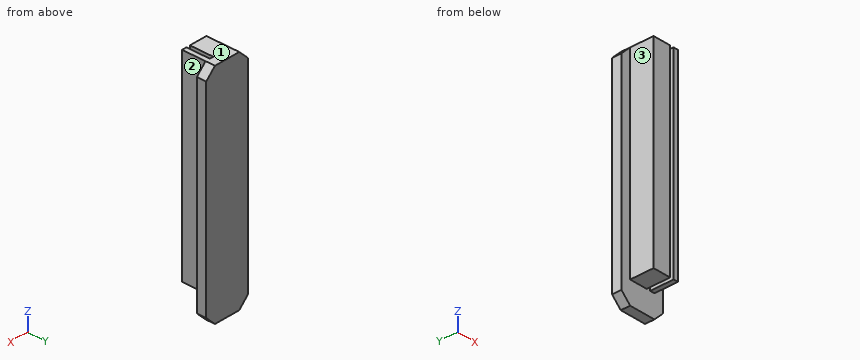
Autodesk Inventor part; units mm, degrees
ref_plane "YZ Plane" through (0, 0, 0) normal (1, 0, 0) x (0, 1, 0)
ref_plane "XZ Plane" through (0, 0, 0) normal (0, 1, 0) x (-1, 0, 0)
ref_plane "XY Plane" through (0, 0, 0) normal (0, 0, 1) x (1, 0, 0)
sketch "Sketch1" plane through (0, 0, 0) normal (0, 1, 0) x (-1, 0, 0)
  line L0 (45.4816, -24) -> (64.4816, -24)
  line L1 (64.4816, -224) -> (45.4816, -224)
  line L2 (64.4816, -24) -> (52.9072, -24)
  line L3 (45.4816, -51) -> (64.4816, -51)
  line L4 (64.4816, -50.2724) -> (64.4816, -24)
  line L5 (64.4816, -69) -> (45.4816, -69)
  line L6 (45.4816, -51) -> (45.4816, -24)
  line L7 (64.4816, -24) -> (64.4816, -51)
  line L8 (64.4816, -154) -> (45.4816, -154)
  line L9 (64.4816, -204) -> (45.4816, -204)
  line L10 (45.4816, -224) -> (45.4816, -204)
  line L11 (45.4816, -154) -> (45.4816, -69)
  line L12 (64.4816, -69) -> (64.4816, -154)
  line L13 (64.4816, -204) -> (64.4816, -224)
  line L14 (41.4816, -24) -> (36.4816, -24)
  line L15 (36.4816, -24) -> (36.4816, -224)
  line L16 (36.4816, -224) -> (41.4816, -224)
  line L17 (41.4816, -224) -> (41.4816, -24)
  point P0 (0, 0)
  dimension "d0" = 200
  dimension "d1" = 19
  dimension "d7" = 27
  dimension "d9" = 45
  dimension "d11" = 85
  dimension "d12" = 20
  dimension "d13" = 4
  dimension "d14" = 19
  dimension "d15" = 5
extrude "Extrusion2" add sketch "Sketch1" along normal blind 11
sketch "Sketch2" plane through (0, 11, 0) normal (0, 1, 0) x (1, 0, 0)
  line L0 (-64.4816, 224) -> (-36.4816, 224)
  line L1 (-36.4816, 224) -> (-36.4816, 24)
  line L2 (-36.4816, 24) -> (-64.4816, 24)
  line L3 (-64.4816, 24) -> (-64.4816, 224)
  point P0 (0, 0)
extrude "Extrusion3" add sketch "Sketch2" along normal blind 3
sketch "Sketch3" plane through (0, 0, 0) normal (0, -1, 0) x (1, 0, 0)
  line L0 (-19.3539, -51.0239) -> (-76.8291, -51.0239)
  line L1 (-76.8291, -51.0239) -> (-76.8291, -110.8451)
  line L2 (-76.8291, -110.8451) -> (-19.3539, -110.8451)
  line L3 (-19.3539, -110.8451) -> (-19.3539, -51.0239)
  line L4 (-25.2187, -135.4773) -> (-86.9948, -135.4773)
  line L5 (-86.9948, -135.4773) -> (-86.9948, -203.9002)
  line L6 (-86.9948, -203.9002) -> (-25.2187, -203.9002)
  line L7 (-25.2187, -203.9002) -> (-25.2187, -135.4773)
  point P0 (0, 0)
extrude "Extrusion4" cut sketch "Sketch3" against normal up to surface (11 mm away)
sketch "Sketch4" plane through (0, 14, 0) normal (0, 1, 0) x (1, 0, 0)
  line L0 (-64.4816, 24) -> (-36.4816, 24)
  line L1 (-26.4816, 34) -> (-26.4816, 251)
  line L2 (-36.4816, 261) -> (-64.4816, 261)
  line L3 (-74.4816, 251) -> (-74.4816, 34)
  line L4 (-64.4816, 224) -> (-64.4816, 24)
  line L5 (-36.4816, 24) -> (-36.4816, 224)
  line L6 (-36.4816, 224) -> (-64.4816, 224)
  line L7 (-64.4816, 24) -> (-74.4816, 34)
  line L8 (-36.4816, 24) -> (-26.4816, 34)
  line L9 (-64.4816, 261) -> (-74.4816, 251)
  line L10 (-36.4816, 261) -> (-26.4816, 251)
  point P0 (0, 0)
  point P1 (-74.4816, 24)
  point P2 (-26.4816, 261)
  point P3 (-26.4816, 24)
  point P4 (-74.4816, 261)
  dimension "d22" = 10
  dimension "d23" = 10
  dimension "d24" = 37
  dimension "d31" = 10
  dimension "d32" = 10
  dimension "d33" = 10
  dimension "d34" = 10
  dimension "d35" = 10
  dimension "d36" = 10
  dimension "d37" = 10
  dimension "d38" = 10
extrude "Extrusion5" add sketch "Sketch4" along normal blind 21
sketch "Sketch5" plane through (-45.4816, 0, -224) normal (0, 0, -1) x (-1, 0, 0)
  line L0 (-9, 0) -> (-4, 0)
  line L1 (-4, 0) -> (-4, 11)
  line L2 (0, 11) -> (-4, 11)
  line L3 (0, 0) -> (0, 11)
  line L4 (19, 0) -> (0, 0)
  line L5 (19, 0) -> (19, 14)
  line L6 (-9, 14) -> (19, 14)
  line L7 (-9, 0) -> (-9, 14)
  point P0 (-45.4816, 0)
extrude "Extrusion6" add sketch "Sketch5" along normal blind 13
sketch "Sketch6" plane through (0, 11, 0) normal (0, -1, 0) x (1, 0, 0)
  line L0 (-41.4816, -51.0239) -> (-41.4816, -24)
  line L1 (-41.4816, -24) -> (-45.4816, -24)
  line L2 (-45.4816, -24) -> (-45.4816, -51)
  line L3 (-45.4816, -51) -> (-64.4816, -51)
  line L4 (-64.4816, -110.8451) -> (-64.4816, -51)
  line L5 (-64.4816, -110.8451) -> (-45.4816, -110.8451)
  line L6 (-45.4816, -110.8451) -> (-45.4816, -135.4773)
  line L7 (-45.4816, -135.4773) -> (-64.4816, -135.4773)
  line L8 (-64.4816, -204) -> (-64.4816, -135.4773)
  line L9 (-64.4816, -204) -> (-45.4816, -204)
  line L10 (-45.4816, -204) -> (-45.4816, -237)
  line L11 (-41.4816, -237) -> (-45.4816, -237)
  line L12 (-41.4816, -203.9002) -> (-41.4816, -237)
  line L13 (-41.4816, -203.9002) -> (-36.4816, -203.9002)
  line L14 (-36.4816, -135.4773) -> (-36.4816, -203.9002)
  line L15 (-36.4816, -135.4773) -> (-41.4816, -135.4773)
  line L16 (-41.4816, -135.4773) -> (-41.4816, -110.8451)
  line L17 (-41.4816, -110.8451) -> (-36.4816, -110.8451)
  line L18 (-36.4816, -51.0239) -> (-36.4816, -110.8451)
  line L19 (-36.4816, -51.0239) -> (-41.4816, -51.0239)
  point P0 (0, 0)
extrude "Extrusion7" cut sketch "Sketch6" against normal up to surface (3 mm away)
sketch "Sketch7" plane through (0, 14, 0) normal (0, -1, 0) x (1, 0, 0)
  line L0 (-36.4816, -110.8451) -> (-36.4816, -135.4773)
  line L1 (-41.4816, -135.4773) -> (-36.4816, -135.4773)
  line L2 (-41.4816, -110.8451) -> (-41.4816, -135.4773)
  line L3 (-36.4816, -110.8451) -> (-41.4816, -110.8451)
  line L4 (-41.4816, -51.0239) -> (-36.4816, -51.0239)
  line L5 (-41.4816, -24) -> (-41.4816, -51.0239)
  line L6 (-45.4816, -24) -> (-41.4816, -24)
  line L7 (-45.4816, -51) -> (-45.4816, -24)
  line L8 (-64.4816, -51) -> (-45.4816, -51)
  line L9 (-64.4816, -51) -> (-64.4816, -24)
  line L10 (-64.4816, -24) -> (-74.4816, -34)
  line L11 (-74.4816, -34) -> (-74.4816, -251)
  line L12 (-74.4816, -251) -> (-64.4816, -261)
  line L13 (-64.4816, -261) -> (-36.4816, -261)
  line L14 (-36.4816, -261) -> (-26.4816, -251)
  line L15 (-26.4816, -251) -> (-26.4816, -34)
  line L16 (-26.4816, -34) -> (-36.4816, -24)
  line L17 (-36.4816, -24) -> (-36.4816, -51.0239)
  line L18 (-36.4816, -203.9002) -> (-36.4816, -237)
  line L19 (-36.4816, -237) -> (-41.4816, -237)
  line L20 (-41.4816, -203.9002) -> (-41.4816, -237)
  line L21 (-36.4816, -203.9002) -> (-41.4816, -203.9002)
  line L22 (-45.4816, -110.8451) -> (-64.4816, -110.8451)
  line L23 (-45.4816, -135.4773) -> (-45.4816, -110.8451)
  line L24 (-64.4816, -135.4773) -> (-45.4816, -135.4773)
  line L25 (-64.4816, -135.4773) -> (-64.4816, -110.8451)
  line L26 (-45.4816, -204) -> (-64.4816, -204)
  line L27 (-45.4816, -237) -> (-45.4816, -204)
  line L28 (-45.4816, -237) -> (-64.4816, -237)
  line L29 (-64.4816, -237) -> (-64.4816, -204)
  point P0 (0, 0)
extrude "Extrusion8" cut sketch "Sketch7" against normal blind 11
sketch "Sketch8" plane through (-64.4816, 0, -204) normal (0, 0, 1) x (1, 0, 0)
  line L0 (0, 0) -> (0, 25)
  line L1 (19, 0) -> (0, 0)
  line L2 (19, 0) -> (19, 25)
  line L3 (19, 25) -> (0, 25)
  line L4 (0, 0) -> (0, 25)
  line L5 (23, 0) -> (23, 25)
  line L6 (28, 0) -> (23, 0)
  line L7 (28, 25) -> (28, 0)
  line L8 (28, 25) -> (23, 25)
  point P0 (64.4816, 0)
extrude "Extrusion9" add sketch "Sketch8" along normal up to surface (180 mm away)
properties part number "cut platform"
Source: CAD feature listing. Evaluate the final solid. Frame: model axes, mm. Face numbers are marked on the shaded views. A direction names the side the tool comes from. Give positions to 0.01 mm unless a question says otherwise; leave off trailing zeros. Loops run counter-clockwise (first coordinate to the right, second up) from the corner with the lowest first, then second, coordinate; pieces in that order, holes last. Notation, with made-up numbers: (82.25, -28) -> (116.25, -28) arc R15 cw to (116.25, -24) -> close; hole circle Ø7 at (-39, 27). An arc over 180 degrees is marked (long way). Use a Markdown table: item, result. Add a question column.
1) First-contact query: pin 1 (8 mm diameter, centred on y = 4, z = -67, fed in from +X); pin 2 (9.5 mm diameter, centred on x = -59, y = 9, fed in from -Z); pin 3 (10 mm diameter, centred on x = -63, y = 21, fed in from -Z); pin 4 (2 mm diameter, centred on y = 13, z = -82, fed in from -X). Flat tips, straight axial feed; report the tip coordinate or a pass-through.
2) Section query D-D, the plane y = 30. Return the cut outline in (x, z), then the cut area to 3 significant figures.
3) Line query: line 1 along X through (y, z) = (6, -60); line 2 along Y through (x, z) = (-40, -250); line 3 along Z through (x, y) = (-47.5, 22.5). Output: solid intervals per line, ascending. Write a range as [from, to].
4) Reachability of the marked faces 1, 2 and 3 from +Z, -Z, +X, -X, +Y, -Y: full face, straight path, thin tool, end or side. Return the list, or none.
5) Section query C-C, the plane x = -60. Return the cut outline in (y, z), then the cut area to 4 significant figures.
6) Section query A-A, the plane y = 4. Return the cut outline in (x, z), then the cut area to 3 significant figures.
7) Section query B-B, the plane z = -147.5. Return the cut outline in (x, y), then the cut area to 3 significant figures.
Numbers:
| question | item | result |
|---|---|---|
| 1 | pin 1 | stops at x = -36.48 |
| 1 | pin 2 | stops at z = -237 |
| 1 | pin 3 | stops at z = -261 |
| 1 | pin 4 | stops at x = -64.48 |
| 2 | outline | (-74.48, -251) -> (-64.48, -261) -> (-36.48, -261) -> (-26.48, -251) -> (-26.48, -34) -> (-36.48, -24) -> (-64.48, -24) -> (-74.48, -34) -> close |
| 2 | area | 11,200 mm2 |
| 3 | line 1 | x = [-64.48, -45.48], [-41.48, -36.48] |
| 3 | line 2 | y = [25, 35] |
| 3 | line 3 | z = [-237, -24] |
| 4 | face 1 | +Z, +X, -X, +Y, -Y |
| 4 | face 2 | +Z, -Z, +X, -Y |
| 4 | face 3 | +Z, -Z, -X, -Y |
| 5 | outline | (0, -237) -> (25, -237) -> (25, -261) -> (35, -261) -> (35, -24) -> (0, -24) -> close |
| 5 | area | 7,695 mm2 |
| 6 | outline | (-64.48, -237) -> (-45.48, -237) -> (-45.48, -24) -> (-64.48, -24) -> close; (-41.48, -237) -> (-36.48, -237) -> (-36.48, -24) -> (-41.48, -24) -> close |
| 6 | area | 5,110 mm2 |
| 7 | outline | (-74.48, 25) -> (-64.48, 25) -> (-64.48, 0) -> (-45.48, 0) -> (-45.48, 25) -> (-41.48, 25) -> (-41.48, 0) -> (-36.48, 0) -> (-36.48, 25) -> (-26.48, 25) -> (-26.48, 35) -> (-74.48, 35) -> close |
| 7 | area | 1,080 mm2 |
